The listing builds one solid part. Answer for the finished solid, in the listing's coordinates (mm). Coordinates: 2 decimals unless noted, no trailing zeros. Order: outer loops, then holes, each group sorted by start corner. A loop starts at its lowest first (then second) coordinate and runs counter-clockwise, first axis right, second up.
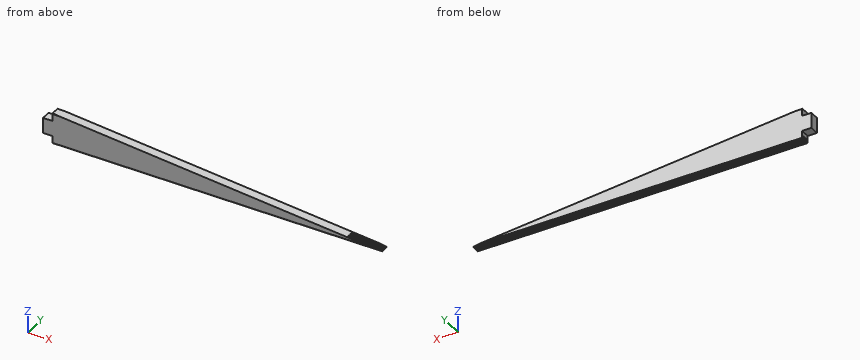
```python
from build123d import *

# Parameters (mm, degrees)
F1_W     = 40
F1_H     = 33
F3_DEPTH = 1275
F2_W     = 80
F2_H     = 100
F4_DEPTH = 25
F6_DEPTH = 50


with BuildPart() as f3:
    # F1 (on Right) → F3 (new body, symmetric)
    with BuildSketch(Plane.YZ):
        Polygon((20, 33), (20, 63), (17, 66), (12, 66), (12, 80), (4, 80), (4, 66), (-4, 66), (-4, 80), (-12, 80), (-12, 66), (-17, 66), (-20, 63), (-20, 33), align=None)
        with Locations((0, 16.5)):
            Rectangle(F1_W, F1_H)
        with Locations((0, -16.5)):
            Rectangle(F1_W, F1_H)
        Polygon((20, -63), (20, -33), (-20, -33), (-20, -63), (-17, -66), (-12, -66), (-12, -52), (-4, -52), (-4, -66), (4, -66), (4, -52), (12, -52), (12, -66), (17, -66), align=None)
    extrude(amount=F3_DEPTH, both=True)

    # F2 (on Front) → F4 (cut, symmetric)
    with BuildSketch(Plane.XZ):
        with Locations((-1275, 83)):
            Rectangle(F2_W, F2_H)
        with Locations((-1275, -83)):
            Rectangle(F2_W, F2_H)
        with Locations((1275, 83)):
            Rectangle(F2_W, F2_H)
        with Locations((1275, -83)):
            Rectangle(F2_W, F2_H)
    extrude(amount=F4_DEPTH, both=True, mode=Mode.SUBTRACT)

    # F5 (on face) → F6 (cut, symmetric)
    with BuildSketch(Plane.XZ.offset(20)):
        Polygon((1525, 88.4753859), (-1475, 88.4753859), (-1202.9649549421, 63), (1235, 63), (1235, 33), (1275, 33), (1275, -33), (1235, -33), (1235, -63), (142.5069374912, -63), (1525, -192.4669378497), align=None)
        Polygon((1235, 63), (-1202.9649549421, 63), (142.5069374912, -63), (1235, -63), (1235, -33), (1275, -33), (1275, 33), (1235, 33), align=None)
    extrude(amount=F6_DEPTH, both=True, mode=Mode.SUBTRACT)


solid = f3.part
```
(1) Find section A-A (x = -790). Write down the section's boundary in (y, z), and give its area (3 significant figures).
(2) Each of these flat-tipped pins is pushed along its axis until it touches: pin 1 Ø3 at (x, y) = (-996, 9.5) entering from -Z; pin 2 Ø6.5 at (x, y) = (-833, 9.5) entering from -Z; pin 3 Ø16.5 at (y, z) = (-5.5, -57.5) entering from -X. Where does it stop, or does it pass through?
(3) Find section B-B (z = 6.5). Write down the section's boundary in (x, y).
(4) Find section C-C (x = -980.5). Write down the section's boundary in (y, z).
(5) Consider line 1 (Y direction, x = -347, z = -56.5); line 2 (Z direction, x = -508, y = -10.5); line 3 (Z direction, x = -443, y = -17.5). Determine where each line is inside the solid, lowest interval first.
Findings below:
1. outline: (-20, -63) - (-17, -66) - (-12, -66) - (-12, -52) - (-4, -52) - (-4, -66) - (4, -66) - (4, -52) - (12, -52) - (12, -66) - (17, -66) - (20, -63) - (20, 24.33) - (-20, 24.33) - close
1. area: 3,380 mm2
2. pin 1: stops at z = -52
2. pin 2: stops at z = -66
2. pin 3: stops at x = -1235
3. outline: (-1275, -20) - (-599.64, -20) - (-599.64, 20) - (-1275, 20) - close
4. outline: (-20, -63) - (-17, -66) - (-12, -66) - (-12, -52) - (-4, -52) - (-4, -66) - (4, -66) - (4, -52) - (12, -52) - (12, -66) - (17, -66) - (20, -63) - (20, 42.17) - (-20, 42.17) - close
5. line 1: y = -20 to -12, -4 to 4, 12 to 20
5. line 2: z = -52 to -2.08
5. line 3: z = -65.5 to -8.17
